```python
from build123d import *

# Parameters (mm, degrees)
SKETCH_W        = 93
SKETCH_H        = 81
PAD_DEPTH       = 10
SKETCH001_W     = 78
SKETCH001_H     = 65
POCKET_DEPTH    = 8
SKETCH002_W     = 90
SKETCH002_H     = 78
POCKET001_DEPTH = 5
SKETCH003_W     = 11.5902
SKETCH003_H     = 11
POCKET002_DEPTH = 8
FILLET_R        = 5
FILLET001_R     = 5
SKETCH004_W     = 14.5
SKETCH004_H     = 14.5
POCKET003_DEPTH = 10.001


with BuildPart() as part:
    # Sketch → Pad (new body)
    with BuildSketch(Plane.XY):
        Rectangle(SKETCH_W, SKETCH_H)
    extrude(amount=PAD_DEPTH)

    # Sketch001 → Pocket (cut)
    with BuildSketch(Plane.XY.offset(10)):
        Rectangle(SKETCH001_W, SKETCH001_H)
    extrude(amount=-POCKET_DEPTH, mode=Mode.SUBTRACT)

    # Sketch002 → Pocket001 (cut)
    with BuildSketch(Plane.XY.offset(10)):
        Rectangle(SKETCH002_W, SKETCH002_H)
    extrude(amount=-POCKET001_DEPTH, mode=Mode.SUBTRACT)

    # Sketch003 → Pocket002 (cut)
    with BuildSketch(Plane.XY.offset(10)):
        with Locations((42.744, -23.7601)):
            Rectangle(SKETCH003_W, SKETCH003_H)
    extrude(amount=-POCKET002_DEPTH, mode=Mode.SUBTRACT)

    # Fillet
    fillet_edges = [part.edges().sort_by_distance(p)[0] for p in [
        (45, 39, 7.5),
        (-45, 39, 7.5),
        (45, -39, 7.5),
        (-45, -39, 7.5),
    ]]
    fillet(fillet_edges, radius=FILLET_R)

    # Fillet001
    fillet001_edges = [part.edges().sort_by_distance(p)[0] for p in [
        (46.5, -40.5, 5),
        (-46.5, -40.5, 5),
        (-46.5, 40.5, 5),
        (46.5, 40.5, 5),
    ]]
    fillet(fillet001_edges, radius=FILLET001_R)

    # Sketch004 → Pocket003 (cut, through all)
    with BuildSketch(Plane(origin=(0, 0, 0), x_dir=(1, 0, 0), z_dir=(0, 0, -1))):
        with Locations((-15.25, -0.25)):
            Rectangle(SKETCH004_W, SKETCH004_H)
    extrude(amount=-POCKET003_DEPTH, mode=Mode.SUBTRACT)


solid = part.part
```
Work out the finished part from the listing and answer in its coordinate system (mm). A direction names the side the tool comes from. Give positions to 0.01 mm unless a question says otherwise; leave off trailing zeros. Order: outer loops, then holes, each group sorted by start corner. A loop starts at its lowest first (then second) coordinate and runs counter-clockwise, first axis right, second up. Notation, with made-up numbers: M 8,-30.75 L 23,-30.75 A33 cw 23,0.25 Z; hole C -32.75,62 d3. An arc over 180 degrees is marked long. Return JSON: item names as keys, results as strings.
1) Straight lines are drawn through the part: line 1 along Y through (x, z) = (5, 2.75); line 2 along Y through (x, z) = (13.5, 7.25); line 3 along X through (y, z) = (34, 5.5). For each, find the intervals that lie inside material, in ascending order. Write a range as [from, to].
Resolved:
{"line 1": "[-40.5, -32.5], [32.5, 40.5]", "line 2": "[-40.5, -39], [39, 40.5]", "line 3": "[-46.5, -45], [45, 46.5]"}
2) Section D-D, the plane y = -11 is taken. Write down the section's boundary in (x, z).
Resolved:
{"outline": "M -46.5,0 L 46.5,0 L 46.5,10 L 45,10 L 45,5 L 39,5 L 39,2 L -39,2 L -39,5 L -45,5 L -45,10 L -46.5,10 Z"}
3) For a pull along Y with two mould halves and no side action, classify faces 6 (the flat face through (-46.5, 0, 5)), 7 (the cylindrical face through (45.07, -39, 5.07)), 8 (the flat face through (-22.5, 0, 1)) as +Y half, -Y half, draft (parallel to the pull), parting line (faces both ways), or undercut.
Resolved:
{"face 6": "draft", "face 7": "-Y half", "face 8": "undercut"}
4) Each of these flat-tipped pins is pushed along its axis until it touches: pin 1 (10 mm diameter, centred on x = -22, y = 29.5, fed in from +Z); pin 2 (5 mm diameter, centred on x = -18, y = -24, fed in from +Z). Where does it stop, or does it pass through?
Resolved:
{"pin 1": "z = 5", "pin 2": "z = 2"}
5) Section C-C, the plane z = 1 is taken. Write down the section's boundary in (x, y), plus the area to 3 significant figures.
Resolved:
{"outline": "M -46.5,-35.5 A5 ccw -41.5,-40.5 L 41.5,-40.5 A5 ccw 46.5,-35.5 L 46.5,35.5 A5 ccw 41.5,40.5 L -41.5,40.5 A5 ccw -46.5,35.5 Z; hole M -22.5,-7 L -8,-7 L -8,7.5 L -22.5,7.5 Z", "area": "7,300 mm^2"}
6) Section A-A, the plane y = 1 is taken. Write down the section's boundary in (x, z), plus the area to 3 significant figures.
Resolved:
{"outline": "M -46.5,0 L -22.5,0 L -22.5,2 L -39,2 L -39,5 L -45,5 L -45,10 L -46.5,10 Z; M -8,0 L 46.5,0 L 46.5,10 L 45,10 L 45,5 L 39,5 L 39,2 L -8,2 Z", "area": "217 mm^2"}
7) A tool of negligible diameter and unlimited length cuts with its end or side. For faces 1 (the flat face through (-0.2, 39.2, 10)), 2 (the flat face through (44, -18.26, 4)), 3 (the flat face through (-15, -7, 1)), 4 (the cylindrical face through (-45.07, -39, 5.07)), 5 (the flat face through (-45, 0, 8)), from which of +Z, -Z, +X, -X, +Y, -Y can it reach the whole face along a straight path? Write none if from no direction.
Resolved:
{"face 1": "+Z, +X, -X, +Y, -Y", "face 2": "+Z, +X", "face 3": "+Z, -Z", "face 4": "+Z, -Z, -X, -Y", "face 5": "+Z"}
8) Section B-B, the plane x = -11 is taken. Write down the section's boundary in (y, z), plus the area to 3 significant figures.
Resolved:
{"outline": "M -40.5,0 L -7,0 L -7,2 L -32.5,2 L -32.5,5 L -39,5 L -39,10 L -40.5,10 Z; M 7.5,0 L 40.5,0 L 40.5,10 L 39,10 L 39,5 L 32.5,5 L 32.5,2 L 7.5,2 Z", "area": "196 mm^2"}
